Design review of the part shown in the three views and the two pictorial views. Dimensions are in mm from the part's minimum x, y and z. Give positions to 0.01 mm unless a question says otherwise; leave off trailing zeros. Loops run counter-clockwise (first coordinate to the right, second up) from the corner with the lowest first, then second, coordinate; pieces in that order, holes last. Notation, with made-up numbers: (-33.75, 48.5) - (-12.75, 48.5) arc R20 cw to (-12.75, 57.5) - close; hole circle Ø9 at (-18, 9). An arc over 180 degrees is marked (long way). Use CSV: the item, a comma, the result in double quotes. Start each with the question number.
1. Take a section at C-C on z = 3.75. Give the boundary of the cut face in (x, y), plus the area to 3 significant figures.
2. Wall thickness on line 1 (X direction, y = 34, z = 4); line 2 (Y direction, x = 11.43, z = 4): over which ranges is each line inside the solid? List them lowest first.
3. Mouldability with a two-part tool opening along X and no side actions: class the marked faces 1, 2 and 3 as pulls with the +X half, pulls with the -X half, needs draft (parallel to the pull), parting line crosses it, or undercut.
4. Take a section at B-B on y = 34.29. Give the boundary of the cut face in (x, z), plus the area to 3 significant figures.
5. Take a section at A-A on x = 11.43. Give the boundary of the cut face in (y, z).
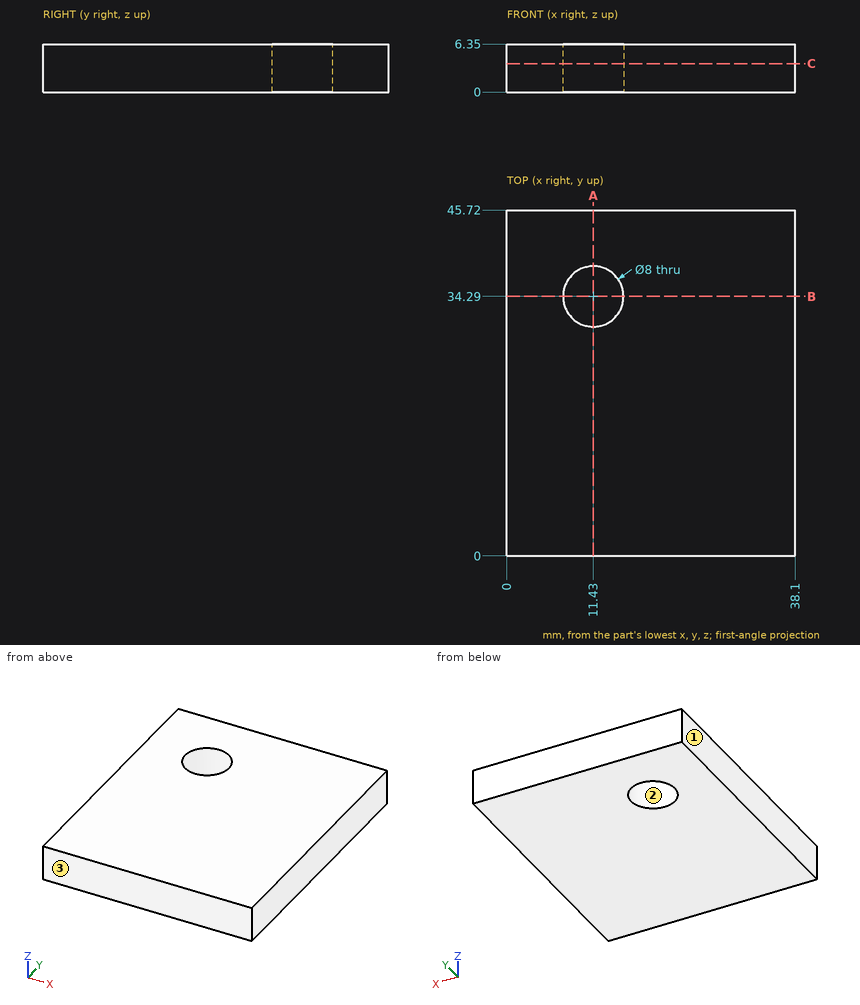
Check result:
1,outline,"(0, 0) - (38.1, 0) - (38.1, 45.72) - (0, 45.72) - close; hole circle Ø8 at (11.43, 34.29)"
1,area,"1,690 mm²"
2,line 1,"x = 0 to 7.44, 15.42 to 38.1"
2,line 2,"y = 0 to 30.29, 38.29 to 45.72"
3,face 1,"pulls with the -X half"
3,face 2,"undercut"
3,face 3,"needs draft"
4,outline,"(0, 0) - (7.43, 0) - (7.43, 6.35) - (0, 6.35) - close; (15.43, 0) - (38.1, 0) - (38.1, 6.35) - (15.43, 6.35) - close"
4,area,"191 mm²"
5,outline,"(0, 0) - (30.29, 0) - (30.29, 6.35) - (0, 6.35) - close; (38.29, 0) - (45.72, 0) - (45.72, 6.35) - (38.29, 6.35) - close"
